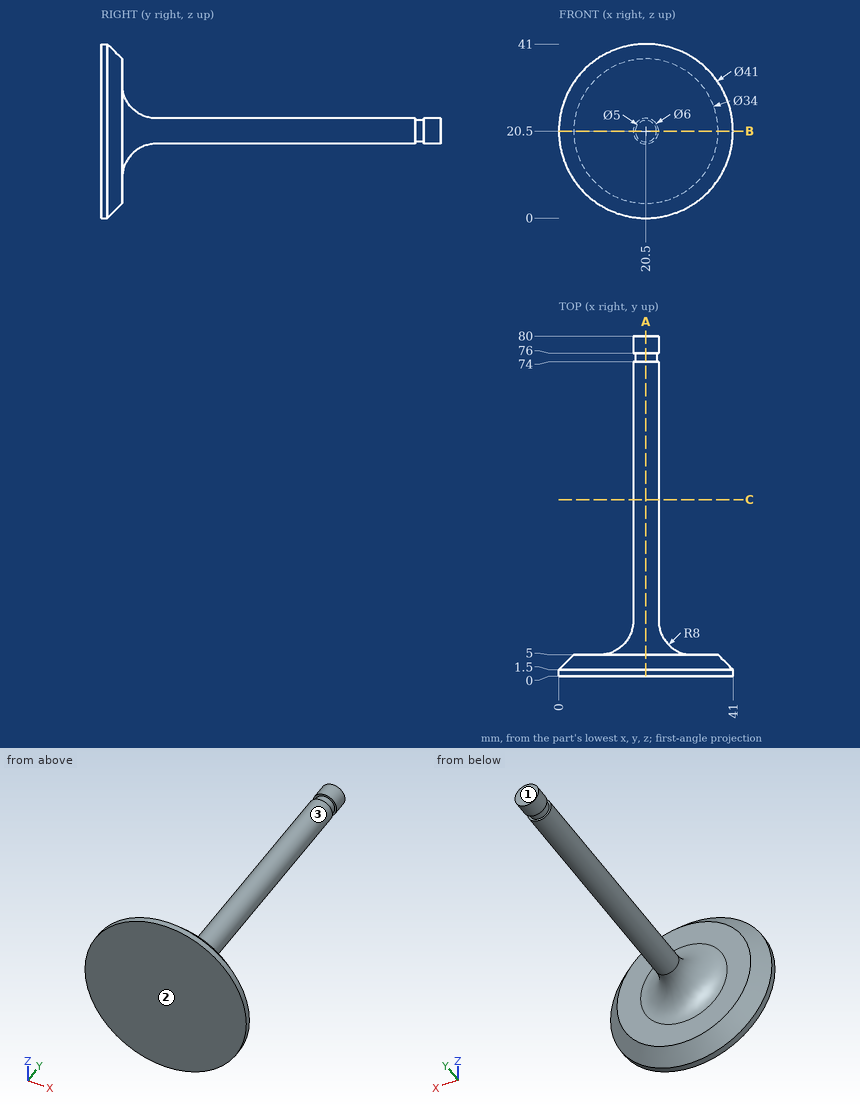
Geometry check sheet. Reference: drawing and pictorial views, mm from the part's lowest x, y, z. Coordinates: 2 decimals unless noted, no trailing zeros. Order: outer loops, then holes, each group sorted by start corner. A loop starts at its lowest first (then second) coordinate and runs counter-clockwise, first axis right, second up. Notation, with made-up numbers: (77.5, -22) -> (134.5, -22) arc R13 ccw to (134.5, 2) -> close; hole circle Ø2 at (47.5, -37.5). An arc over 180 degrees is marked (long way). Write item = value, one per line. Start each with the question number.
1) Go/stop test with flat-tipped pins: P1, Ø8, axis at x = 27, y = 16, coming from the -Z side; P2, Ø10, axis at y = 46.5, z = 26, coming from the -X side; P3, Ø3, axis at x = 24.5, y = 59, coming from the +Z side. Record where each tip stops, or that it passes through.
2) Material ranges on L1, parallel to Y at x = 25, z = 5; L2, parallel to Y at x = 39.5, z = 25.5; L3, parallel to X at y = 20, z = 22, recorded low to high.
3) Cross-section at C-C (y = 41.5). Enter the section's corners in (x, z), then the cut area to 3 significant figures.
4) Mould release check, pull along Y, two halves, no side actions. Record for the marked faces 1, 2 and 3: +Y half, -Y half, draft (parallel to the pull), parting line (faces both ways), or undercut.
5) Cross-section at B-B (z = 20.5). Enter the section's corners in (x, y), then the cut area to 3 significant figures.
6) Cross-section at A-A (x = 20.5). Enter the section's corners in (y, z).
Ans:
q1.P1 = 18.84
q1.P2 = 17.54
q1.P3 = 22.16
q2.L1 = 0 to 5
q2.L2 = 0 to 2.35
q2.L3 = 17.9 to 23.1
q3.outline = circle Ø6 at (20.5, 20.5)
q3.area = 28.3 mm²
q4.face_1 = +Y half
q4.face_2 = -Y half
q4.face_3 = draft
q5.outline = (0, 0) -> (41, 0) -> (41, 1.5) -> (37.5, 5) -> (31.5, 5) arc R8 cw to (23.5, 13) -> (23.5, 74) -> (23, 74) -> (23, 76) -> (23.5, 76) -> (23.5, 80) -> (17.5, 80) -> (17.5, 76) -> (18, 76) -> (18, 74) -> (17.5, 74) -> (17.5, 13) arc R8 cw to (9.5, 5) -> (3.5, 5) -> (0, 1.5) -> close
q5.area = 668 mm²
q6.outline = (0, 0) -> (1.5, 0) -> (5, 3.5) -> (5, 9.5) arc R8 cw to (13, 17.5) -> (74, 17.5) -> (74, 18) -> (76, 18) -> (76, 17.5) -> (80, 17.5) -> (80, 23.5) -> (76, 23.5) -> (76, 23) -> (74, 23) -> (74, 23.5) -> (13, 23.5) arc R8 cw to (5, 31.5) -> (5, 37.5) -> (1.5, 41) -> (0, 41) -> close
